Verification items for the finished model (mm, model axes). Coordinates: 2 decimals unless noted, no trailing zeros. Write each loop counter-clockwise with the first axis right and the second up, starting at its lowest first coordinate (ties: lowest second). Pieces come first, ordered by that corner, then holes. Notation, with made-up numbers: (0.25, 52) -> (9.25, 52) arc R37 cw to (9.25, 89) -> close; hole circle Ø8 at (-8.75, -28.75). An arc over 180 degrees is marked (long way). Answer in a Markdown table with one row per item.
Autodesk Inventor part; units mm, degrees
ref_plane "YZ Plane" through (0, 0, 0) normal (1, 0, 0) x (0, 1, 0)
ref_plane "XZ Plane" through (0, 0, 0) normal (0, 1, 0) x (-1, 0, 0)
ref_plane "XY Plane" through (0, 0, 0) normal (0, 0, 1) x (1, 0, 0)
sketch "Sketch1" plane through (0, 0, 0) normal (0, 1, 0) x (-1, 0, 0)
  line L0 (4, 10) -> (-19.4211, 10)
  line L1 (-19.4211, -10) -> (4, -10)
  line L2 (4, -10) -> (4, 10)
  arc A0 (-19.4211, -10) -> (-19.4211, 10) centre (-25.1, 0) ccw
  line L3 (4, -10) -> (6, -10)
  line L4 (6, -10) -> (6, 10)
  line L5 (6, 10) -> (4, 10)
  line L6 (4, 10) -> (4, -10)
  point P0 (0, 0)
  dimension "d0" = 20
  dimension "d2" = 4
  dimension "d3" = 10
  dimension "d6" = 10
  dimension "d7" = 23
  dimension "d8" = 29.1
  dimension "d11" = 23.4211
  dimension "d12" = 20
  dimension "d13" = 2
extrude "Extrusion1" add sketch "Sketch1" along normal blind 6.61
fillet "Fillet1" radius 1 2 edges at (19.4211, 3.305, -10) (19.4211, 3.305, 10)
sketch "Sketch3" plane through (0, 0, 0) normal (0, -1, 0) x (1, 0, 0)
  circle A0 centre (-2.5, -7.525) radius 1.05
  circle A1 centre (12.6, -7.525) radius 1.05
  circle A2 centre (12.6, 7.525) radius 1.05
  circle A3 centre (-2.5, 7.525) radius 1.05
  point P0 (0, 0)
hole "Hole2" at (-2.5, 0, -7.525) at (-2.5, 0, 7.525) at (12.6, 0, 7.525) at (12.6, 0, -7.525) direction (0, 1, 0) diameter 2.1 end through all
sketch "Sketch4" plane through (0, 0, 0) normal (0, -1, 0) x (1, 0, 0)
  line L0 (1.4953, 17.8846) -> (19.0725, -12.5601)
  arc A0 (17.1193, 8.28) -> (17.1193, -8.28) centre (25.1, 0) ccw
  arc A1 (17.1193, 8.28) -> (16.4253, 10) centre (16.4253, 9) ccw
  line L1 (-6, 10) -> (16.4253, 10)
  point P0 (0, 0)
  point P1 (6.0474, 10)
  point P2 (15.1407, -5.75)
  dimension "d29" = 60
extrude "Extrusion2" cut sketch "Sketch4" against normal up to next
properties part number "3D_printed_part"
1. Material ranges on probe 1 along Z at (x, y) = (-2.5, 4.25) (3 decimals); probe 2 along Z at (x, y) = (-3, 3); probe 3 along X at (y, z) = (1.5, 8), recorded low to high. Write a range as from..to.
Findings below:
| item | result |
|---|---|
| probe 1 | z = -10..-8.575, -6.475..6.475, 8.575..10 |
| probe 2 | z = -10..-8.45, -6.6..6.6, 8.45..10 |
| probe 3 | x = -6..-3.44, -1.56..7.2 |
2. Go/stop test with flat-tipped pins: pin 1 (1.5 mm diameter, centred on x = 9, y = 2, fed in from +Z); pin 2 (3 mm diameter, centred on y = 3.5, z = -3, fed in from +X). Record where each tip stops, or that it passes through.
Findings below:
| item | result |
|---|---|
| pin 1 | stops at z = 6.19 |
| pin 2 | stops at x = 14.42 |
3. Sectioned sample at B-B, the plane x = -2.5. Record the cut outline in (y, z) (3 decimals).
Findings below:
| item | result |
|---|---|
| outline | (0, -10) -> (6.61, -10) -> (6.61, -8.575) -> (0, -8.575) -> close; (0, -6.475) -> (6.61, -6.475) -> (6.61, 6.475) -> (0, 6.475) -> close; (0, 8.575) -> (6.61, 8.575) -> (6.61, 10) -> (0, 10) -> close |
4. Release check for a two-part mould opening along Z. For faces 1 (the face through (3, 0, -2)), 2 (the face through (-3.385, 3.351, -8.089)), 3 (the face through (0, 3, 10)), 4 (the face through (17.36, 3.35, -9.36)) record: released by +Z, released by -Z, zero draft, split by the parting line, or undercut.
Findings below:
| item | result |
|---|---|
| face 1 | zero draft |
| face 2 | undercut |
| face 3 | released by +Z |
| face 4 | split by the parting line |
5. Sectioned sample at C-C, the plane z = -7.25. Record the cut outline in (x, y).
Findings below:
| item | result |
|---|---|
| outline | (-6, 0) -> (-3.51, 0) -> (-3.51, 6.61) -> (-6, 6.61) -> close; (-1.49, 0) -> (11.59, 0) -> (11.59, 6.61) -> (-1.49, 6.61) -> close; (13.61, 0) -> (16.17, 0) -> (16.17, 6.61) -> (13.61, 6.61) -> close |
6. Sectioned sample at D-D, the plane x = 12.6. Record the cut outline in (y, z) (3 decimals), and give its area (3 significant figures).
Findings below:
| item | result |
|---|---|
| outline | (0, -10) -> (6.61, -10) -> (6.61, -8.575) -> (0, -8.575) -> close; (0, -6.475) -> (6.61, -6.475) -> (6.61, -1.349) -> (0, -1.349) -> close |
| area | 43.3 mm² |
7. Sectioned sample at A-A, the plane y = 4. Record the cut outline in (x, z) (3 decimals).
Findings below:
| item | result |
|---|---|
| outline | (-6, -10) -> (16.425, -10) arc R1 ccw to (17.119, -8.28) arc R11.5 cw to (15.141, -5.75) -> (6.047, 10) -> (-6, 10) -> close; hole circle Ø2.1 at (-2.5, -7.525); hole circle Ø2.1 at (-2.5, 7.525); hole circle Ø2.1 at (12.6, -7.525) |
